The listing builds one solid part. Answer for the finished solid, in the listing's coordinates (mm). A direction names the side the tool comes from. Coordinates: 2 decimals unless noted, no trailing zeros. Write each loop counter-clockwise with the first axis right and the second up, starting at its lowest first coordinate (ties: lowest second). Pieces come first, ordered by that corner, then holes.
from build123d import *

# Parameters (mm, degrees)
EXTRUDE_1_DEPTH     = 3.5
SKETCH_4_R          = 8.79
SKETCH_4_R_2        = 4
CUT_EXTRUDE_1_DEPTH = 0.4375
CUT_EXTRUDE_1_DRAFT = -60
CHAMFER_2_SIZE      = 0.277777778
SKETCH_9_W          = 7
SKETCH_9_H          = 5
CUT_EXTRUDE_2_DEPTH = 5


with BuildPart() as part:
    # 草图3 → 凸台-拉伸1 (new body)
    with BuildSketch(Plane(origin=(0, 0, 0), x_dir=(0, 0, -1), z_dir=(1, 0, 0))):
        Polygon((4, 2.309401077), (0, 4.618802154), (-4, 2.309401077), (-4, -2.309401077), (0, -4.618802154), (4, -2.309401077), align=None)
    extrude(amount=EXTRUDE_1_DEPTH)


with BuildPart() as cut_extrude_1_tool:
    # 草图4 → 切除-拉伸1 (with draft: the straight prism first)
    with BuildSketch(Plane.ZY):
        Circle(SKETCH_4_R)
        Circle(SKETCH_4_R_2, mode=Mode.SUBTRACT)
    extrude(amount=-CUT_EXTRUDE_1_DEPTH)
    # 切除-拉伸1: the draft: its side faces are tilted about the plane it starts from
    cut_extrude_1_sides = [cut_extrude_1_tool.faces().sort_by_distance(p)[0] for p in [
        (0.21875, 0, -8.79),
        (0.21875, 0, -4),
    ]]
    draft(cut_extrude_1_sides, Plane.ZY, CUT_EXTRUDE_1_DRAFT)


with BuildPart() as part_1:
    add(part.part)

    # 切除-拉伸1: cut by cut_extrude_1_tool
    add(cut_extrude_1_tool.part, mode=Mode.SUBTRACT)

    # 草图5 → 旋转1 (revolve)
    with BuildSketch(Plane.XY, mode=Mode.PRIVATE) as revolve_1_sk:
        with BuildLine():
            Line((3.85, 2.5), (13.5, 2.5))
            Line((13.5, 2.5), (13.5, 0))
            Line((13.5, 0), (3.5, 0))
            Line((3.5, 0), (3.5, 2.85))
            ThreePointArc((3.5, 2.85), (3.602512627, 2.602512627), (3.85, 2.5))
        make_face()
    revolve(revolve_1_sk.sketch.rotate(Axis((3.5, 0, 0), (1, 0, 0)), 90), axis=Axis((3.5, 0, 0), (1, 0, 0)))

    # 倒角2
    chamfer_2_edges = [part_1.edges().sort_by_distance(p)[0] for p in [
        (13.5, 0, -2.5),
    ]]
    chamfer(chamfer_2_edges, length=CHAMFER_2_SIZE)

    # 草图7 → 切除-旋转1 (revolve, cut)
    with BuildSketch(Plane.XY, mode=Mode.PRIVATE) as cut_revolve_1_sk:
        Polygon((3.5, 3.34), (3, 3.84), (3, 8.79), (3.5, 8.79), align=None)
    revolve(cut_revolve_1_sk.sketch.rotate(Axis((0, 0, 0), (1, 0, 0)), 90), axis=Axis((0, 0, 0), (1, 0, 0)), mode=Mode.SUBTRACT)

    # 草图9 → 切除-拉伸2 (cut, symmetric)
    with BuildSketch(Plane.XY):
        with Locations((13.5, 0)):
            Rectangle(SKETCH_9_W, SKETCH_9_H)
    extrude(amount=CUT_EXTRUDE_2_DEPTH, both=True, mode=Mode.SUBTRACT)


solid = part_1.part
1. Find the intervals of material crossed by L1, parallel to X at y = -3.25, z = 0.5; L2, parallel to Z at x = 5.75, y = 1.5; L3, parallel to Y at x = 6.25, z = -1.25, in increasing order.
Results found:
L1: x = 0 to 3.5
L2: z = -2 to 2
L3: y = -2.17 to 2.17
2. Flat-ended cylindrical pins translate along their axes: P1, Ø1, axis at x = 8.5, z = -1.5, coming from the -Y side; P2, Ø5, axis at x = 5, y = 2.5, coming from the -Z side. Find the tip coordinate at first contact, or state that the pin passes through.
Results found:
P1: stops at y = -2.29
P2: stops at z = -4
3. Section B-B on x = 7.5 is taken. Give the vertices of the cut face in (y, z), then the cut area to 3 significant figures.
Results found:
outline: circle Ø5 at (0, 0)
area: 19.6 mm2
4. Section A-A on x = 0.75 is taken. Give the vertices of the cut face in (y, z), then the cut area to 3 significant figures.
Results found:
outline: (-4.62, 0) - (-2.31, -4) - (2.31, -4) - (4.62, 0) - (2.31, 4) - (-2.31, 4) - close
area: 55.4 mm2
5. A tool of negligible diameter and unlimited length cuts with its end or side. For faces 1 (the flat face through (3.5, 1, -3)), 2 (the flat face through (10, 0, 0)), from which of +Z, -Z, +X, -X, +Y, -Y can it reach the whole face along a straight path? Write none if from no direction.
Results found:
face 1: +X
face 2: +Z, -Z, +X, +Y, -Y
